```python
from build123d import *

# Parameters (mm, degrees)
ESTRUSIONE_ESTRUSIONE1_DEPTH = 5.6


with BuildPart() as part:
    # Schizzo1 → Estrusione-Estrusione1 (new body)
    with BuildSketch(Plane.XY):
        Polygon((-17.425, 53.416651246), (-17.425, 56.291651246), (-22.575, 56.291651246), (-22.575, 53.416651246), (-27.425, 53.416651246), (-27.425, 56.291651246), (-32.5, 56.291651246), (-35.0375, 51.896572322), (-32.547676964, 50.459072322), (-34.972676964, 46.258849113), (-37.4625, 47.696349113), (-40.0375, 43.236318284), (-37.547676964, 41.798818284), (-39.972676964, 37.598595076), (-42.4625, 39.036095076), (-45.0375, 34.576064246), (-42.547676964, 33.138564246), (-44.972676964, 28.938341038), (-47.4625, 30.375841038), (-50.0375, 25.915810208), (-47.547676964, 24.478310208), (-49.972676964, 20.278087), (-52.4625, 21.715587), (-55.0375, 17.25555617), (-52.547676964, 15.81805617), (-54.972676964, 11.617832962), (-57.4625, 13.055332962), (-60.0375, 8.595302133), (-57.547676964, 7.157802133), (-59.972676964, 2.957578924), (-62.4625, 4.395078924), (-65, 0), (-62.4625, -4.395078924), (-59.972676964, -2.957578924), (-57.547676964, -7.157802133), (-60.0375, -8.595302133), (-57.4625, -13.055332962), (-54.972676964, -11.617832962), (-52.547676964, -15.81805617), (-55.0375, -17.25555617), (-52.4625, -21.715587), (-49.972676964, -20.278087), (-47.547676964, -24.478310208), (-50.0375, -25.915810208), (-47.4625, -30.375841038), (-44.972676964, -28.938341038), (-42.547676964, -33.138564246), (-45.0375, -34.576064246), (-42.4625, -39.036095076), (-39.972676964, -37.598595076), (-37.547676964, -41.798818284), (-40.0375, -43.236318284), (-37.4625, -47.696349113), (-34.972676964, -46.258849113), (-32.547676964, -50.459072322), (-35.0375, -51.896572322), (-32.5, -56.291651246), (-27.425, -56.291651246), (-27.425, -53.416651246), (-22.575, -53.416651246), (-22.575, -56.291651246), (-17.425, -56.291651246), (-17.425, -53.416651246), (-12.575, -53.416651246), (-12.575, -56.291651246), (-7.425, -56.291651246), (-7.425, -53.416651246), (-2.575, -53.416651246), (-2.575, -56.291651246), (2.575, -56.291651246), (2.575, -53.416651246), (7.425, -53.416651246), (7.425, -56.291651246), (12.575, -56.291651246), (12.575, -53.416651246), (17.425, -53.416651246), (17.425, -56.291651246), (22.575, -56.291651246), (22.575, -53.416651246), (27.425, -53.416651246), (27.425, -56.291651246), (32.5, -56.291651246), (35.0375, -51.896572322), (32.547676964, -50.459072322), (34.972676964, -46.258849113), (37.4625, -47.696349113), (40.0375, -43.236318284), (37.547676964, -41.798818284), (39.972676964, -37.598595076), (42.4625, -39.036095076), (45.0375, -34.576064246), (42.547676964, -33.138564246), (44.972676964, -28.938341038), (47.4625, -30.375841038), (50.0375, -25.915810208), (47.547676964, -24.478310208), (49.972676964, -20.278087), (52.4625, -21.715587), (55.0375, -17.25555617), (52.547676964, -15.81805617), (54.972676964, -11.617832962), (57.4625, -13.055332962), (60.0375, -8.595302133), (57.547676964, -7.157802133), (59.972676964, -2.957578924), (62.4625, -4.395078924), (65, 0), (62.4625, 4.395078924), (59.972676964, 2.957578924), (57.547676964, 7.157802133), (60.0375, 8.595302133), (57.4625, 13.055332962), (54.972676964, 11.617832962), (52.547676964, 15.81805617), (55.0375, 17.25555617), (52.4625, 21.715587), (49.972676964, 20.278087), (47.547676964, 24.478310208), (50.0375, 25.915810208), (47.4625, 30.375841038), (44.972676964, 28.938341038), (42.547676964, 33.138564246), (45.0375, 34.576064246), (42.4625, 39.036095076), (39.972676964, 37.598595076), (37.547676964, 41.798818284), (40.0375, 43.236318284), (37.4625, 47.696349113), (34.972676964, 46.258849113), (32.547676964, 50.459072322), (35.0375, 51.896572322), (32.5, 56.291651246), (27.425, 56.291651246), (27.425, 53.416651246), (22.575, 53.416651246), (22.575, 56.291651246), (17.425, 56.291651246), (17.425, 53.416651246), (12.575, 53.416651246), (12.575, 56.291651246), (7.425, 56.291651246), (7.425, 53.416651246), (2.575, 53.416651246), (2.575, 56.291651246), (-2.575, 56.291651246), (-2.575, 53.416651246), (-7.425, 53.416651246), (-7.425, 56.291651246), (-12.575, 56.291651246), (-12.575, 53.416651246), align=None)
    extrude(amount=ESTRUSIONE_ESTRUSIONE1_DEPTH)


solid = part.part
```
Geometry: final body of the model. Coordinates: model frame, mm. A direction names the side the tool comes from. Coordinates: 2 decimals unless noted, no trailing zeros. Answer in a Markdown table with one row per item. Add a question column.
Q1. Contact query for flat-ended pins moving along their axis: P1, Ø2.5, axis at y = -55, z = 2, coming from the -X side; P2, Ø1.4, axis at y = -54.5, z = 2, coming from the -X side; P3, Ø2, axis at y = -41.5, z = 4.5, coming from the -X side; P4, Ø2, axis at x = -16.5, z = 3, coming from the +Y side. Output: stop coordinate, or through.
Q2. Mould query, pull axis X, two halves, no side actions, for faces 1 (the flat face through (0, -56.292, 3)), 2 (the flat face through (53.77, 19.45, 2.76)), 3 (the flat face through (-48.74, 22.41, 2.76)). Classes: released by +X, released by -X, zero draft, split by the parting line, or undercut.
Q3. Line query: L1, parallel to Y at x = -54, z = 1.95; L2, parallel to Y at x = 44, z = 4.9; L3, parallel to Y at x = -47, z = 0.5. Output: solid intervals per line, ascending.
Q4. Reachability of faces 4 (the flat face through (-33.74, 48.39, 2.76)), 5 (the flat face through (-27.425, 55, 3)), 6 (the flat face through (-30, -56.292, 3)) from +Z, -Z, +X, -X, +Y, -Y: full face, straight path, thin tool, end or side. Return the list, or none.
Completed:
| question | item | result |
|---|---|---|
| 1 | P1 | stops at x = -33.97 |
| 1 | P2 | stops at x = -33.94 |
| 1 | P3 | stops at x = -38.76 |
| 1 | P4 | stops at y = 56.29 |
| 2 | face 1 | zero draft |
| 2 | face 2 | released by +X |
| 2 | face 3 | undercut |
| 3 | L1 | y = -19.05 to -16.66, -13.3 to 13.3, 16.66 to 19.05 |
| 3 | L2 | y = -36.37 to -33.98, -30.62 to 30.62, 33.98 to 36.37 |
| 3 | L3 | y = -30.11 to 30.11 |
| 4 | face 4 | +Z, -Z |
| 4 | face 5 | +Z, -Z, +Y |
| 4 | face 6 | +Z, -Z, +X, -X, -Y |
